Source: CAD feature listing. Evaluate the final solid. Frame: model axes, mm. Face numbers are marked on the shaded views. A direction names the side the tool comes from. Round coordinates to 2 decimals unless told otherwise and drop trailing zeros. Loops run counter-clockwise (first coordinate to the right, second up) from the corner with the lowest first, then second, coordinate; pieces in that order, holes last.
(1) Mould query, pull axis X, two halves, no side actions, for the marked faces 1, 2 and 3. Classes: pulls with the +X half, pulls with the -X half, needs draft (parallel to the pull), parting line crosses it, or undercut.
(2) Section D-D, the plane y = 20.5. Return the cut outline in (x, z), plus the area to 3 significant figures.
(3) Section B-B, the plane x = 14. Return the cut outline in (y, z).
(4) Section C-C, the plane y = -13. Return the cut outline in (x, z), plus the area to 3 significant figures.
(5) Set-up query: the marked faces 4 and 5. Return all of +Z, -Z, +X, -X, +Y, -Y with unobstructed straight access to the full face (end or side cutting, diameter ignored); none if empty.
(6) Section A-A, the plane y = 0.5. Return the cut outline in (x, z).
(7) First-contact query: pin 1 Ø3 at (x, y) = (7.5, 0.5) entering from +Z; pin 2 Ø2 at (x, y) = (-51, 16.5) entering from +Z; pin 3 Ø3 at (x, z) = (-54.5, 10) entering from +Y; pin 4 Ø2 at (x, y) = (-55, -1) entering from -Z. Flat tips, straight axial feed; report the tip coordinate or a pass-through.
(8) Material intervals for probe 1 along Y at (x, z) = (-51.5, 6.5); probe 2 along Y at (x, z) = (-35.5, 5); probe 3 along X at (y, z) = (-21.5, 4.75), sorted ascending.
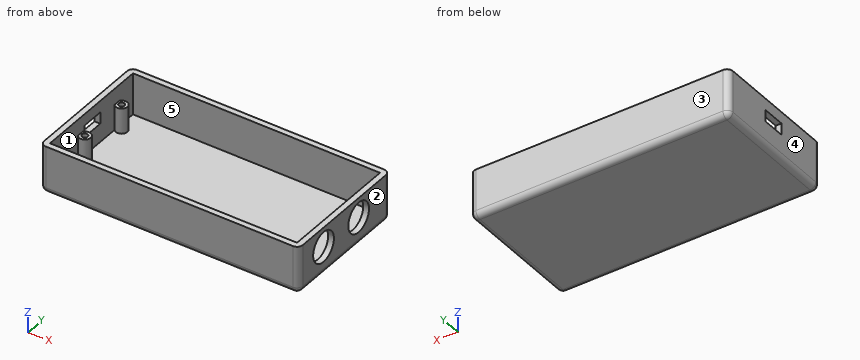
```python
from build123d import *

# Parameters (mm, degrees)
SKETCH_W        = 107
SKETCH_H        = 52
PAD_DEPTH       = 18
THICKNESS_T     = 2.5
SKETCH001_R     = 6.5
POCKET_DEPTH    = 5
SKETCH002_W     = 10
SKETCH002_H     = 5
POCKET001_DEPTH = 5
SKETCH003_R     = 2.5
SKETCH003_R_2   = 1.25
PAD001_DEPTH    = 11


with BuildPart() as part:
    # Sketch → Pad (new body)
    with BuildSketch(Plane.XY):
        Rectangle(SKETCH_W, SKETCH_H)
    extrude(amount=PAD_DEPTH)

    # Thickness
    thickness_openings = [part.faces().sort_by_distance(p)[0] for p in [
        (0, 0, 18),
    ]]
    offset(amount=THICKNESS_T, openings=thickness_openings)

    # Sketch001 (on DatumPlane) → Pocket (cut)
    with BuildSketch(Plane(origin=(53.5, 0, 0), x_dir=(0, -1, 0), z_dir=(-1, 0, 0))):
        with Locations((-9, 9.5)):
            Circle(SKETCH001_R)
        with Locations((13, 9.5)):
            Circle(SKETCH001_R)
    extrude(amount=-POCKET_DEPTH, mode=Mode.SUBTRACT)

    # Sketch002 (on DatumPlane) → Pocket001 (cut)
    with BuildSketch(Plane.YZ.offset(-53.5)):
        with Locations((0.5, 10.5)):
            Rectangle(SKETCH002_W, SKETCH002_H)
    extrude(amount=-POCKET001_DEPTH, mode=Mode.SUBTRACT)

    # Sketch003 (on DatumPlane) → Pad001 (join)
    with BuildSketch(Plane.XY):
        with Locations((-51.5, 16)):
            Circle(SKETCH003_R)
        with Locations((-51.5, 16)):
            Circle(SKETCH003_R_2, mode=Mode.SUBTRACT)
        with Locations((-51.5, -7)):
            Circle(SKETCH003_R)
        with Locations((-51.5, -7)):
            Circle(SKETCH003_R_2, mode=Mode.SUBTRACT)
    extrude(amount=PAD001_DEPTH)


solid = part.part
```
Output values:
1. face 1: undercut
1. face 2: pulls with the +X half
1. face 3: needs draft
2. outline: (-56, 0) arc R2.5 ccw to (-53.5, -2.5) - (53.5, -2.5) arc R2.5 ccw to (56, 0) - (56, 18) - (53.5, 18) - (53.5, 0) - (-53.5, 0) - (-53.5, 18) - (-56, 18) - close
2. area: 367 mm2
3. outline: (-28.5, 0) arc R2.5 ccw to (-26, -2.5) - (26, -2.5) arc R2.5 ccw to (28.5, 0) - (28.5, 18) - (26, 18) - (26, 0) - (-26, 0) - (-26, 18) - (-28.5, 18) - close
4. outline: (-56, 0) arc R2.5 ccw to (-53.5, -2.5) - (53.5, -2.5) arc R2.5 ccw to (56, 0) - (56, 3) - (53.5, 3) - (53.5, 0) - (-53.5, 0) - (-53.5, 18) - (-56, 18) - close; (53.5, 16) - (56, 16) - (56, 18) - (53.5, 18) - close
4. area: 335 mm2
5. face 4: +Z, -Z, -X, +Y, -Y
5. face 5: +Z
6. outline: (-56, 0) arc R2.5 ccw to (-53.5, -2.5) - (53.5, -2.5) arc R2.5 ccw to (56, 0) - (56, 18) - (53.5, 18) - (53.5, 0) - (-53.5, 0) - (-53.5, 8) - (-56, 8) - close; (-56, 13) - (-53.5, 13) - (-53.5, 18) - (-56, 18) - close
7. pin 1: stops at z = 0
7. pin 2: stops at z = 11
7. pin 3: stops at y = 28.5
7. pin 4: stops at z = -2.45
8. probe 1: y = -28.5 to -26, -9.5 to -8.25, -5.75 to -4.5, 13.5 to 14.75, 17.25 to 18.5, 26 to 28.5
8. probe 2: y = -28.5 to -26, 26 to 28.5
8. probe 3: x = -56 to -53.5, 53.5 to 56
